Input: part model. Units: mm. Frame: model coordinates. Face numbers are marked on the shaded views. A direction names the side the tool comes from. Give positions to 0.01 mm unless a question says otherwise; leave off trailing zeros. Loops run counter-clockwise (first coordinate to the right, second up) from the corner with the lowest first, then second, coordinate; pieces in that order, holes last. Notation, with made-up numbers: (29, 35.25) - (74, 35.25) arc R19 ccw to (74, 55.25) - close; hole circle Ø7 at (27, 2.5). An arc over 180 degrees is marked (long way). Answer as a JSON object with one key per item and string values.
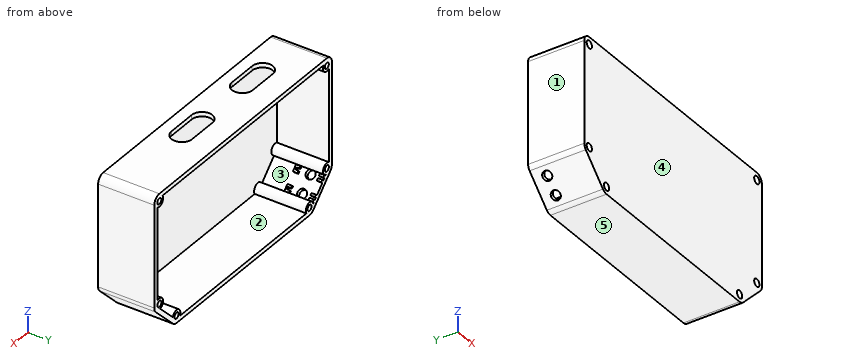
from build123d import *

# Parameters (mm, degrees)
BOSS_EXTRUDE1_DEPTH = 3
BOSS_EXTRUDE2_DEPTH = 35
SKETCH3_R           = 3.1
CUT_EXTRUDE1_DEPTH  = 10
SKETCH4_W           = 1.5
SKETCH4_H           = 3
BOSS_EXTRUDE3_DEPTH = 1.5
SKETCH6_R           = 3.75
BOSS_EXTRUDE4_DEPTH = 35
SKETCH7_R           = 2
CUT_EXTRUDE2_DEPTH  = 38
SKETCH8_R           = 2.6
CUT_EXTRUDE3_DEPTH  = 25
CUT_EXTRUDE4_DEPTH  = 3
FILLET1_R           = 5


with BuildPart() as part:
    # Sketch1 → Boss-Extrude1 (new body)
    with BuildSketch(Plane(origin=(0, 0, 0), x_dir=(1, 0, 0), z_dir=(0, 1, 0))):
        Polygon((-68, 48), (-88, 28), (-88, -48), (88, -48), (88, 28), (68, 48), align=None)
    extrude(amount=BOSS_EXTRUDE1_DEPTH)

    # Sketch2 → Boss-Extrude2 (add)
    with BuildSketch(Plane(origin=(0, 3, 0), x_dir=(1, 0, 0), z_dir=(0, 1, 0))):
        Polygon((88, 28), (68, 48), (-68, 48), (-88, 28), (-88, -48), (88, -48), align=None)
        Polygon((85, -45), (85, 26.757359313), (66.757359313, 45), (-66.757359313, 45), (-85, 26.757359313), (-85, -45), align=None, mode=Mode.SUBTRACT)
    extrude(amount=BOSS_EXTRUDE2_DEPTH)

    # Sketch3 → Cut-Extrude1 (cut)
    with BuildSketch(Plane(origin=(-58, 0, -58), x_dir=(-0.7071067811865475, 0, 0.7071067811865477), z_dir=(-0.7071067811865477, 0, -0.7071067811865475))):
        with Locations((34.284271247, 29)):
            Circle(SKETCH3_R)
        with Locations((22.284271247, 29)):
            Circle(SKETCH3_R)
    extrude(amount=-CUT_EXTRUDE1_DEPTH, mode=Mode.SUBTRACT)

    # Sketch4 → Boss-Extrude3 (add)
    with BuildSketch(Plane(origin=(-55.878679656, 0, -55.878679656), x_dir=(0.7071067811865476, 0, -0.7071067811865475), z_dir=(0.7071067811865475, 0, 0.7071067811865476))):
        with Locations((-20.834271247, 36.5)):
            Rectangle(SKETCH4_W, SKETCH4_H)
        Polygon((-22.284271247, 18.8), (-22.284271247, 19.8), (-22.984271247, 19.8), (-22.984271247, 21.8), (-24.484271247, 21.8), (-24.484271247, 18.8), align=None)
        Polygon((-21.584271247, 19.8), (-22.284271247, 19.8), (-22.284271247, 18.8), (-20.084271247, 18.8), (-20.084271247, 21.8), (-21.584271247, 21.8), align=None)
        Polygon((-32.084271247, 18.8), (-32.084271247, 21.8), (-33.584271247, 21.8), (-33.584271247, 19.8), (-34.984271247, 19.8), (-34.984271247, 21.8), (-36.484271247, 21.8), (-36.484271247, 18.8), align=None)
        with Locations((-35.734271247, 36.5)):
            Rectangle(SKETCH4_W, SKETCH4_H)
        with Locations((-23.734271247, 36.5)):
            Rectangle(SKETCH4_W, SKETCH4_H)
        with Locations((-32.834271247, 36.5)):
            Rectangle(SKETCH4_W, SKETCH4_H)
    extrude(amount=BOSS_EXTRUDE3_DEPTH)

    # Sketch6 → Boss-Extrude4 (add)
    with BuildSketch(Plane(origin=(0, 3, 0), x_dir=(1, 0, 0), z_dir=(0, 1, 0))):
        with Locations((-65.928932188, 43)):
            Circle(SKETCH6_R)
        with Locations((65.928932188, 43)):
            Circle(SKETCH6_R)
        with Locations((83, 25.928932188)):
            Circle(SKETCH6_R)
        with Locations((83, -43)):
            Circle(SKETCH6_R)
        with Locations((-83, -43)):
            Circle(SKETCH6_R)
        with Locations((-83, 25.928932188)):
            Circle(SKETCH6_R)
    extrude(amount=BOSS_EXTRUDE4_DEPTH)

    # Sketch7 → Cut-Extrude2 (cut)
    with BuildSketch(Plane(origin=(0, 38, 0), x_dir=(1, 0, 0), z_dir=(0, 1, 0))):
        with Locations(Location((-65.928932188, 43, 0), (0, 0, 270))):
            Circle(SKETCH7_R)
        with Locations(Location((-83, 25.928932188, 0), (0, 0, 270))):
            Circle(SKETCH7_R)
        with Locations(Location((-83, -43, 0), (0, 0, 270))):
            Circle(SKETCH7_R)
        with Locations(Location((83, -43, 0), (0, 0, 270))):
            Circle(SKETCH7_R)
        with Locations(Location((83, 25.928932188, 0), (0, 0, 270))):
            Circle(SKETCH7_R)
        with Locations(Location((65.928932188, 43, 0), (0, 0, 270))):
            Circle(SKETCH7_R)
    extrude(amount=-CUT_EXTRUDE2_DEPTH, mode=Mode.SUBTRACT)

    # Sketch8 → Cut-Extrude3 (cut)
    with BuildSketch(Plane.XZ):
        with Locations(Location((-83, 43, 0), (0, 0, 270))):
            Circle(SKETCH8_R)
        with Locations(Location((83, 43, 0), (0, 0, 270))):
            Circle(SKETCH8_R)
        with Locations(Location((83, -25.928932188, 0), (0, 0, 270))):
            Circle(SKETCH8_R)
        with Locations(Location((65.928932188, -43, 0), (0, 0, 270))):
            Circle(SKETCH8_R)
        with Locations(Location((-65.928932188, -43, 0), (0, 0, 270))):
            Circle(SKETCH8_R)
        with Locations(Location((-83, -25.928932188, 0), (0, 0, 270))):
            Circle(SKETCH8_R)
    extrude(amount=-CUT_EXTRUDE3_DEPTH, mode=Mode.SUBTRACT)

    # Sketch9 → Cut-Extrude4 (cut)
    with BuildSketch(Plane.XY.offset(48)):
        with BuildLine():
            Line((-33, 8), (-53, 8))
            ThreePointArc((-53, 8), (-60, 15), (-53, 22))
            Line((-53, 22), (-33, 22))
            ThreePointArc((-33, 22), (-26, 15), (-33, 8))
        make_face()
        with BuildLine():
            Line((27, 8), (7, 8))
            ThreePointArc((7, 8), (0, 15), (7, 22))
            Line((7, 22), (27, 22))
            ThreePointArc((27, 22), (34, 15), (27, 8))
        make_face()
    extrude(amount=-CUT_EXTRUDE4_DEPTH, mode=Mode.SUBTRACT)

    # Fillet1
    fillet1_edges = [part.edges().sort_by_distance(p)[0] for p in [
        (88, 19, 48),
        (-88, 19, 48),
        (-88, 19, -28),
        (-68, 19, -48),
        (68, 19, -48),
        (88, 19, -28),
    ]]
    fillet(fillet1_edges, radius=FILLET1_R)


solid = part.part
Item 1: Cut plane D-D (x = 53). Return loops of the section in (y, z), then the cut area to 3 significant figures.
Geometry check:
{"outline": "(0, -48) - (38, -48) - (38, -45) - (3, -45) - (3, 45) - (38, 45) - (38, 48) - (0, 48) - close", "area": "498 mm2"}
Item 2: Mould query, pull axis Y, two halves, no side actions, for the marked faces 3, 4 and 5. Classes: released by +Y, released by -Y, zero draft, split by the parting line, or undercut.
Geometry check:
{"face 3": "undercut", "face 4": "released by -Y", "face 5": "zero draft"}
Item 3: Access query for the marked faces 1 and 2. Directions: +Z, -Z, +X, -X, +Y, -Y. A direction counts if a zero-diameter tool reaches every point of the face in a straight line with its end or side. Return the directions, or none.
Geometry check:
{"face 1": "+Z, -Z, -X, +Y, -Y", "face 2": "+Y"}
Item 4: Cut plane A-A (x = 18). Return loops of the section in (y, z).
Geometry check:
{"outline": "(0, -48) - (38, -48) - (38, -45) - (3, -45) - (3, 45) - (8, 45) - (8, 48) - (0, 48) - close; (22, 45) - (38, 45) - (38, 48) - (22, 48) - close"}
Item 5: Contact query for flat-ended pins moving along their axis: P1, Ø4.5, axis at x = -65.93, z = -43, coming from the -Y side; P2, Ø3, axis at x = 83, z = -25.93, coming from the -Y side; P3, Ø0.6, axis at x = -71, z = -40, coming from the +Y side; P4, Ø8, axis at y = 22, z = -37, coming from the -X side. Output: stop coordinate, or through.
Geometry check:
{"P1": "stops at y = 25", "P2": "passes through", "P3": "stops at y = 19.8", "P4": "stops at x = -83"}
Item 6: Material intervals for line 1 (X direction, y = 8.5, z = 43); line 2 (X direction, y = 35, z = 43); line 3 (X direction, y = 25, z = 12), sorted ascending. Write a range as [from, to].
Geometry check:
{"line 1": "x = [-88, -85.6], [-80.4, -79.25], [79.25, 80.4], [85.6, 88]", "line 2": "x = [-88, -85], [-81, -79.25], [79.25, 81], [85, 88]", "line 3": "x = [-88, -85], [85, 88]"}
Item 7: Cut plane B-B (y = 15). Give the number of separate pieces and of enclosed holes in the cut face, then the cut area to 3 significant figures.
Geometry check:
{"separate pieces": "2", "enclosed holes": "6", "area": "1,370 mm2"}
Item 8: Cut plane C-C (z = 10). Return loops of the section in (x, y).
Geometry check:
{"outline": "(-88, 0) - (88, 0) - (88, 38) - (85, 38) - (85, 3) - (-85, 3) - (-85, 38) - (-88, 38) - close"}
